```python
from build123d import *

# Parameters (mm, degrees)
ESBO_O1_W                = 50
ESBO_O1_H                = 50
RESSALTO_EXTRUS_O1_DEPTH = 28
ESBO_O2_W                = 45
ESBO_O2_H                = 47.5
CORTE_EXTRUS_O1_DEPTH    = 28
ESBO_O3_R                = 5
CORTE_EXTRUS_O2_DEPTH    = 63.521996129
ESBO_O4_R                = 5
CORTE_EXTRUS_O3_DEPTH    = 63.521996129
FILETE1_R                = 14


with BuildPart() as part:
    # Esboço1 → Ressalto-extrusão1 (new body)
    with BuildSketch(Plane.XY):
        Rectangle(ESBO_O1_W, ESBO_O1_H)
    extrude(amount=RESSALTO_EXTRUS_O1_DEPTH)

    # Esboço2 → Corte-extrusão1 (cut)
    with BuildSketch(Plane(origin=(0, 0, 0), x_dir=(-1, 0, 0), z_dir=(0, 0, -1))):
        with Locations((0, -1.25)):
            Rectangle(ESBO_O2_W, ESBO_O2_H)
    extrude(amount=-CORTE_EXTRUS_O1_DEPTH, mode=Mode.SUBTRACT)

    # Esboço3 → Corte-extrusão2 (cut, through all)
    with BuildSketch(Plane(origin=(0, 25, 0), x_dir=(1, 0, 0), z_dir=(0, 1, 0))):
        with Locations(Location((0, -14, 0), (0, 0, 270))):
            Circle(ESBO_O3_R)
    extrude(amount=-CORTE_EXTRUS_O2_DEPTH, mode=Mode.SUBTRACT)

    # Esboço4 → Corte-extrusão3 (cut, through all)
    with BuildSketch(Plane(origin=(25, 0, 0), x_dir=(0, 0, -1), z_dir=(1, 0, 0))):
        with Locations(Location((-14, -11, 0), (0, 0, 90))):
            Circle(ESBO_O4_R)
    extrude(amount=-CORTE_EXTRUS_O3_DEPTH, mode=Mode.SUBTRACT)

    # Filete1
    filete1_edges = [part.edges().sort_by_distance(p)[0] for p in [
        (23.75, -25, 28),
        (-23.75, -25, 28),
        (-23.75, -25, 0),
        (23.75, -25, 0),
    ]]
    fillet(filete1_edges, radius=FILETE1_R - 0.0001)  # a hair under: the kernel refuses the full size


solid = part.part
```
Geometry: final body of the model. Coordinates: model frame, mm. A direction names the side the tool comes from. Round coordinates to 2 decimals unless told otherwise and drop trailing zeros. Order: outer loops, then holes, each group sorted by start corner. A loop starts at its lowest first (then second) coordinate and runs counter-clockwise, first axis right, second up. Notation, with made-up numbers: (60, 87.5) -> (80, 87.5) arc R24 cw to (80, 110.5) -> close; hole circle Ø7 at (47.5, 80.5). An arc over 180 degrees is marked (long way). Use one line per item in the form item = value. Start each with the question number.
1. Cut plane D-D (z = 6.5). Return the cut outline in (x, y).
2. Cut plane B-B (x = 0). Return the cut outline in (y, z), then the cut area to 3 significant figures.
3. Cut plane C-C (z = 15.5). Return the cut outline in (x, y).
4. Reachability of faces 1 (the face through (23.8, -20.8, 24)), 2 (the face through (5.3, 22.5, 13.8)) from +Z, -Z, +X, -X, +Y, -Y: full face, straight path, thin tool, end or side. Return the list, or none.
5. Pin query (flat end, axial travel): pin 1 Ø1.5 at (x, z) = (-5.5, 15.5) entering from -Y. Return the tip coordinate at first contact, or that it passes through.
6. Cut plane A-A (y = 7). Return the cut outline in (x, z).
7. Draft query along X for faces 3 (the face through (23.8, -20.8, 4)), 4 (the face through (25, 0, 14)), 5 (the face through (22.5, -2, 14)). Return one class per face: pulls with the +X half, pulls with the -X half, needs draft (parallel to the pull), parting line crosses it, or undercut.
8. Line query: probe 1 along X at (y, z) = (23.5, 14); probe 2 along X at (y, z) = (-19, 19.5); probe 3 along Z at (x, y) = (-23, -11). Output: solid intervals per line, ascending.
Solution:
q1.outline = (-25, -22.82) -> (-22.5, -22.82) -> (-22.5, 22.5) -> (22.5, 22.5) -> (22.5, -22.82) -> (25, -22.82) -> (25, 25) -> (-25, 25) -> close
q2.outline = (22.5, 0) -> (25, 0) -> (25, 9) -> (22.5, 9) -> close; (22.5, 19) -> (25, 19) -> (25, 28) -> (22.5, 28) -> close
q2.area = 45.0 mm^2
q3.outline = (-25, -24.92) -> (-22.5, -24.92) -> (-22.5, -15.77) -> (-25, -15.77) -> close; (-25, -6.23) -> (-22.5, -6.23) -> (-22.5, 22.5) -> (-4.77, 22.5) -> (-4.77, 25) -> (-25, 25) -> close; (4.77, 22.5) -> (22.5, 22.5) -> (22.5, -6.23) -> (25, -6.23) -> (25, 25) -> (4.77, 25) -> close; (22.5, -24.92) -> (25, -24.92) -> (25, -15.77) -> (22.5, -15.77) -> close
q4.face_1 = +Z, +X, -X, -Y
q4.face_2 = +Z, -Z, -Y
q5.pin_1 = 22.5
q6.outline = (-25, 0) -> (-22.5, 0) -> (-22.5, 28) -> (-25, 28) -> close; (22.5, 0) -> (25, 0) -> (25, 28) -> (22.5, 28) -> close
q7.face_3 = needs draft
q7.face_4 = pulls with the +X half
q7.face_5 = undercut
q8.probe_1 = -25 to -5, 5 to 25
q8.probe_2 = -25 to -22.5, 22.5 to 25
q8.probe_3 = 0 to 9, 19 to 28
